The drawing under review shows one solid part. Ordinate dimensions are in mm from its lowest x, y, z. A direction names the side the tool comes from. Give positions to 0.01 mm unless a question says otherwise; leave off trailing zeros. Write each loop counter-clockwise with the first axis right and the second up, starting at its lowest first coordinate (ties: lowest second). Pieces come first, ordered by that corner, then holes. Notation, with made-up numbers: (42, 75) - (93, 75) arc R17 ccw to (93, 94) - close; hole circle Ø9 at (34.5, 36). An arc over 180 degrees is marked (long way). Write item = value, one per line.
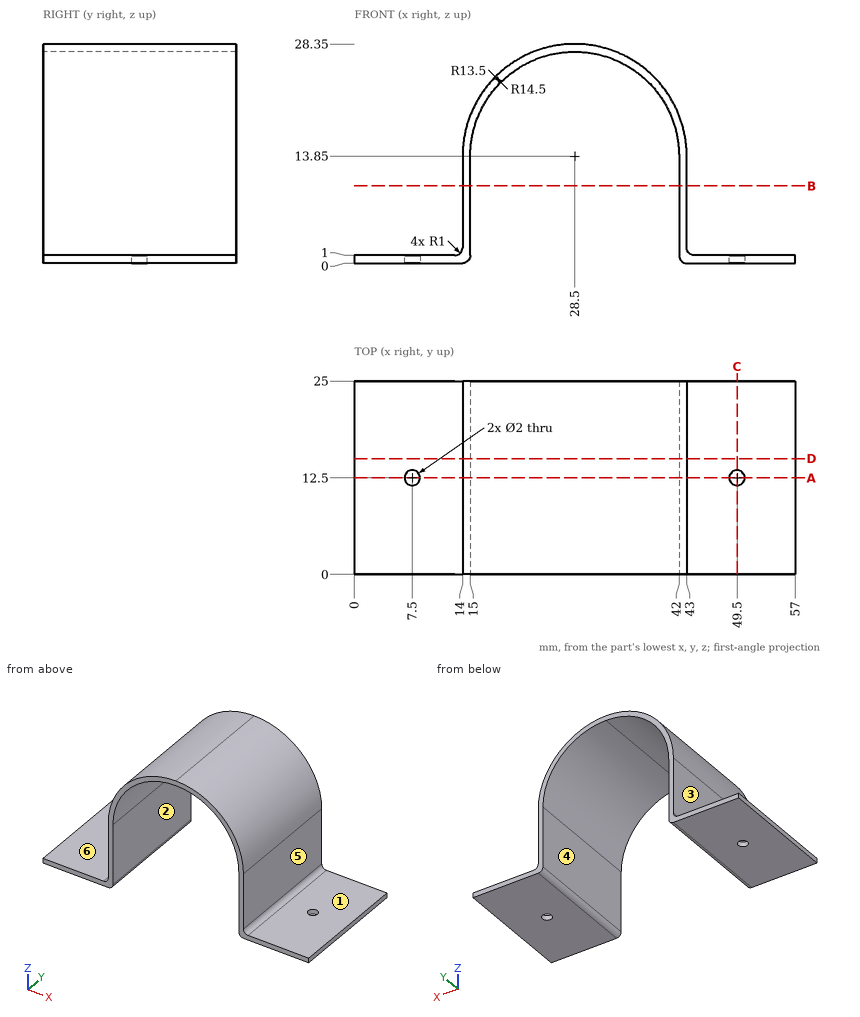
1. For line 1 (Y direction, x = 49.5, z = 0.4); line 2 (X direction, y = 2, z = 11.75); line 3 (Z direction, x = 51, y = 16.75), list the stretches that pass through material, from the lowest coordinate up. Write a range as from..to.
Findings below:
line_1 = 0..11.5, 13.5..25
line_2 = 14..15, 42..43
line_3 = 0..1
2. Take a section at A-A on y = 12.5. Give the boundary of the cut face in (x, z), and give its area (3 significant figures).
Findings below:
outline = (0, 0) - (6.5, 0) - (6.5, 1) - (0, 1) - close; (8.5, 0) - (14, 0) arc R1 ccw to (15, 1) - (15, 13.85) arc R13.5 cw to (28.5, 27.35) arc R13.5 cw to (42, 13.85) - (42, 1) arc R1 ccw to (43, 0) - (48.5, 0) - (48.5, 1) - (44, 1) arc R1 cw to (43, 2) - (43, 13.85) arc R14.5 ccw to (28.5, 28.35) arc R14.5 ccw to (14, 13.85) - (14, 2) arc R1 cw to (13, 1) - (8.5, 1) - close; (50.5, 0) - (57, 0) - (57, 1) - (50.5, 1) - close
area = 95.7 mm²
3. Take a section at C-C on x = 49.5. Give the boundary of the cut face in (y, z).
Findings below:
outline = (0, 0) - (11.5, 0) - (11.5, 1) - (0, 1) - close; (13.5, 0) - (25, 0) - (25, 1) - (13.5, 1) - close
4. Take a section at D-D on y = 15. Give the boundary of the cut face in (x, z).
Findings below:
outline = (0, 0) - (14, 0) arc R1 ccw to (15, 1) - (15, 13.85) arc R13.5 cw to (28.5, 27.35) arc R13.5 cw to (42, 13.85) - (42, 1) arc R1 ccw to (43, 0) - (57, 0) - (57, 1) - (44, 1) arc R1 cw to (43, 2) - (43, 13.85) arc R14.5 ccw to (28.5, 28.35) arc R14.5 ccw to (14, 13.85) - (14, 2) arc R1 cw to (13, 1) - (0, 1) - close
5. Draft analysis for pull direction X (two halves, no side actions). For the marked faces 1, 2 and 3, state which applies: +X half, -X half, draft (parallel to the pull), parting line (faces both ways), or undercut.
Findings below:
face_1 = draft
face_2 = undercut
face_3 = -X half
6. Insertion check: P1, Ø6.5, axis at x = 7.5, y = 10.5, coming from the +Z side; P2, Ø12, axis at y = 16.5, z = 12.5, coming from the +X side; P3, Ø6, axis at y = 6, z = 25, coming from the -X side; P4, Ø3, axis at x = 30.5, z = 24, coming from the +Y side. Each pin has a flat end and moves straight along its axis. Give the tip position at first contact, or say it passes through.
Findings below:
P1 = 1
P2 = 43
P3 = 16.51
P4 = through
7. Machinability: for the marked faces 4, 5 and 6, which of the approach directions +Z, -Z, +X, -X, +Y, -Y give a long, thin tool a straight path to every point of the face, cutting with its end or side? Answer none if there is none.
Findings below:
face_4 = -Z, +Y, -Y
face_5 = +Z, +X, +Y, -Y
face_6 = +Z, -X, +Y, -Y
8. Take a section at B-B on z = 10. Give the boundary of the cut face in (x, y), and give its area (3 significant figures).
Findings below:
outline = (14, 0) - (15, 0) - (15, 25) - (14, 25) - close; (42, 0) - (43, 0) - (43, 25) - (42, 25) - close
area = 50.0 mm²
